Autodesk Inventor part; units mm, degrees
ref_plane "Work Plane2" through (2.032, 0, 0) normal (0, 1, 0) x (1, 0, 0)
ref_plane "YZ Plane" through (0, 0, 0) normal (1, 0, 0) x (0, 1, 0)
ref_plane "XZ Plane" through (0, 0, 0) normal (0, 1, 0) x (-1, 0, 0)
sketch "Sketch1" plane through (0, 0, 0) normal (0, 0, 1) x (1, 0, 0)
  line L0 (1.6002, 0) -> (6.35, 0)
  line L1 (6.35, 0) -> (6.35, 1.2573)
  line L2 (6.35, 1.2573) -> (1.0922, 1.2573)
  line L3 (0.3676, 2.1209) -> (0, 2.1209)
  line L4 (-1.27, 0) -> (7.62, 0)
  line L5 (0, -0.4242) -> (0, 2.5451)
  line L6 (0, 1.2954) -> (1.2402, 0.6771)
  line L7 (1.2402, 0.6771) -> (1.6002, 0)
  line L8 (1.0922, 1.2573) -> (0.3676, 2.1209)
  line L9 (0, 2.1209) -> (0, 1.2954)
  dimension "d2" = 2.5146
  dimension "d3" = 4.2418
  dimension "d4" = 1.6002
  dimension "d5" = 2.5908
  dimension "d6" = 26.5
  dimension "d7" = 62
  dimension "d13" = 50
  dimension "d14" = 1.0922
  dimension "d15" = 6.35
revolve "Body" add sketch "Sketch1" angle 360 about axis through (1.6002, 0, 0) along (1, 0, 0) contours L7 L6 L5 L3 L8 L2 L1 L0
sketch "Sketch2" plane through (0, 0, 0) normal (-1, 0, 0) x (0, 0, 1)
  line L0 (0, -2.9693) -> (0, 2.9693)
  line L1 (-2.9693, 0) -> (2.9693, 0)
  line L2 (0, 1.2954) -> (0, 0) construction
  line L3 (0, 0) -> (1.2954, 0) construction
  arc A0 (0.4318, 0) -> (0, 0.4318) centre (0, 0) ccw
  line L4 (0, 0) -> (0.7947, 0.7947) construction
  arc A1 (0.6477, 0) -> (0, 0.6477) centre (0, 0) ccw construction
  line L5 (0.1778, 1.2831) -> (0.1744, 0.6238)
  line L6 (1.2831, 0.1778) -> (0.6238, 0.1744)
  arc A2 (0.1744, 0.6238) -> (0.6238, 0.1744) centre (0.6215, 0.6215) ccw
  arc A3 (1.2954, 0) -> (1.2831, 0.1778) centre (0, 0) ccw
  arc A4 (0.1778, 1.2831) -> (0, 1.2954) centre (0, 0) ccw
  arc A5 (1.2831, 0.1778) -> (0.1778, 1.2831) centre (0, 0) ccw
  line L7 (0.1778, -1.2831) -> (0.1744, -0.6238)
  line L8 (1.2831, -0.1778) -> (0.6238, -0.1744)
  arc A6 (0.6238, -0.1744) -> (0.1744, -0.6238) centre (0.6215, -0.6215) ccw
  arc A7 (1.2831, -0.1778) -> (1.2954, 0) centre (0, 0) ccw
  arc A8 (0, -1.2954) -> (0.1778, -1.2831) centre (0, 0) ccw
  arc A9 (0.1778, -1.2831) -> (1.2831, -0.1778) centre (0, 0) ccw
  line L9 (-0.1778, 1.2831) -> (-0.1744, 0.6238)
  line L10 (-1.2831, 0.1778) -> (-0.6238, 0.1744)
  arc A10 (-0.6238, 0.1744) -> (-0.1744, 0.6238) centre (-0.6215, 0.6215) ccw
  arc A11 (-1.2831, 0.1778) -> (-1.2954, 0) centre (0, 0) ccw
  arc A12 (0, 1.2954) -> (-0.1778, 1.2831) centre (0, 0) ccw
  arc A13 (-0.1778, 1.2831) -> (-1.2831, 0.1778) centre (0, 0) ccw
  arc A14 (-1.2831, -0.1778) -> (-0.1778, -1.2831) centre (0, 0) ccw
  arc A15 (-0.1778, -1.2831) -> (0, -1.2954) centre (0, 0) ccw
  arc A16 (-1.2954, 0) -> (-1.2831, -0.1778) centre (0, 0) ccw
  line L11 (-1.2831, -0.1778) -> (-0.6238, -0.1744)
  arc A17 (-0.1744, -0.6238) -> (-0.6238, -0.1744) centre (-0.6215, -0.6215) ccw
  line L12 (-0.1778, -1.2831) -> (-0.1744, -0.6238)
  dimension "d18" = 45
  dimension "d19" = 0.8636
  dimension "d20" = 1.2954
  dimension "d21" = 2.5908
  dimension "d22" = 0.1778
extrude "Slot" add sketch "Sketch2" against normal up to next contours A2 L5 A5 L6 | L9 A10 L10 A13 | L7 A6 L8 A9 | A14 L11 A17 L12
fillet "Fillet1" radius 0.0711 4 edges at (0, 1.2954, 0) (0, 0, 1.2954) (0, -1.2954, 0) (0, 0, -1.2954)
thread "Thread"
chamfer "Chamfer1" distance 0.3148 distance2 0.3148 1 edges at (6.35, -1.2573, 0) measured on face at (6.35, -0.6343, -0.3329)
ref_plane "Work Plane2" through (2.032, 0, 0) normal (0, 1, 0) x (1, 0, 0)
equation "\"d2\" = GD"
equation "\"d3\" = KOD"
equation "\"d4\" = INTI"
equation "\"d5\" = SDM"
equation "\"d13\" = 0.5 * SEWI"
equation "\"d14\" = KOH"
equation "\"d15\" = NLG"
equation "\"d19\" = 0.333333 * SDM"
equation "\"d20\" = 0.5 * SDM"
equation "\"d21\" = SDM"
equation "\"d22\" = 0.5 * SBR"
equation "\"d45\" = INTI"
equation "\"d25\" = 0.2 * SBR"
equation "\"d9\" = GEL"
equation "\"d11\" = -0.5 * SPD + 0.5 * GD"
equation "\"d12\" = GUL"
equation "\"GD\" = NND"
equation "\"NLG\" = 6.35"
equation "\"GEL\" = 3.9349"
equation "\"KOD\" = 4.2418"
equation "\"KOH\" = 1.0922"
equation "\"SDM\" = 2.5908"
equation "\"INTI\" = 1.6002"
equation "\"SBR\" = 0.3556"
equation "\"GUL\" = -0.5 * SPD + 0.5 * NND"
equation "\"SPD\" = 1.8849"
equation "\"SEWI\" = 100deg"
equation "\"d0\" = NLG"
equation "\"d1\" = KOH"
equation "\"d17\" = SDM"
equation "\"TOA\" = 30deg"
equation "\"EPV\" = 2.1472"
equation "\"THREADDIA\" = 2.5146"
equation "\"BDM\" = NND"
equation "\"NND\" = 2.5146"
equation "\"GAL\" = 0.52916"
equation "\"GD1\" = SPD"
properties part number "ANSI B18.6.3 - 3-48 UNC x 0,25" material "Steel, Mild"
The listing builds one solid part. Answer for the finished solid, in the listing's coordinates (mm). Give positions to 0.01 mm unless a question says otherwise; leave off trailing zeros. Write each loop counter-clockwise with the first axis right and the second up, starting at its lowest first coordinate (ties: lowest second). Pieces come first, ordered by that corner, then holes. Notation, with made-up numbers: (-12.5, 1.5) -> (27.5, 1.5) arc R19 cw to (27.5, 26.5) -> close; hole circle Ø9 at (83, 70). An arc over 180 degrees is marked (long way). One line per question, with ' | ' between items. Start each with the question number.
1. Find the intervals of material crossed by probe 1 along Z at (x, y) = (1, 0.45); probe 2 along Z at (x, y) = (4.5, 0); probe 3 along Y at (x, z) = (0.5, 0.1), in increasing order.
2. For a pull along Z with two mould halves and no side action, classify faces 1 (the flat face through (6.35, 0, 0)), 2 (the conical face through (1.6, 0, 0)), 3 (the cylindrical face through (3.53, -0.27, 1.23)) as pulls with the +Z half, pulls with the -Z half, needs draft (parallel to the pull), parting line crosses it, or undercut.
3. Section A-A (x = 5.25) is taken. Determine the outline of the cut face in (y, z).
Response values:
1) probe 1: -1.29 to -0.21, 0.21 to 1.29 | probe 2: -1.26 to 1.26 | probe 3: -1.96 to -1.04, 1.04 to 1.96
2) face 1: needs draft | face 2: undercut | face 3: parting line crosses it
3) outline: circle Ø2.51 at (0, 0)
